from build123d import *

# Parameters (mm, degrees)
F0_W     = 80
F0_H     = 19
F1_DEPTH = 19
F2_R     = 4
F3_DEPTH = 12
F2_R_2   = 5
F4_DEPTH = 2


with BuildPart() as f1:
    # F0 (on Top) → F1 (new body)
    with BuildSketch(Plane.XY):
        Rectangle(F0_W, F0_H)
    extrude(amount=F1_DEPTH)

    # F2 (on face) → F3 (cut)
    with BuildSketch(Plane(origin=(0, 9.5, 0), x_dir=(-1, 0, 0), z_dir=(0, 1, 0))):
        with Locations((20, 9.5)):
            Circle(F2_R)
        with Locations((-20, 9.5)):
            Circle(F2_R)
    extrude(amount=-F3_DEPTH, mode=Mode.SUBTRACT)

    # F2 (on face) → F4 (cut)
    with BuildSketch(Plane(origin=(0, 9.5, 0), x_dir=(-1, 0, 0), z_dir=(0, 1, 0))):
        with Locations((0, 9.5)):
            Circle(F2_R_2)
    extrude(amount=-F4_DEPTH, mode=Mode.SUBTRACT)


solid = f1.part
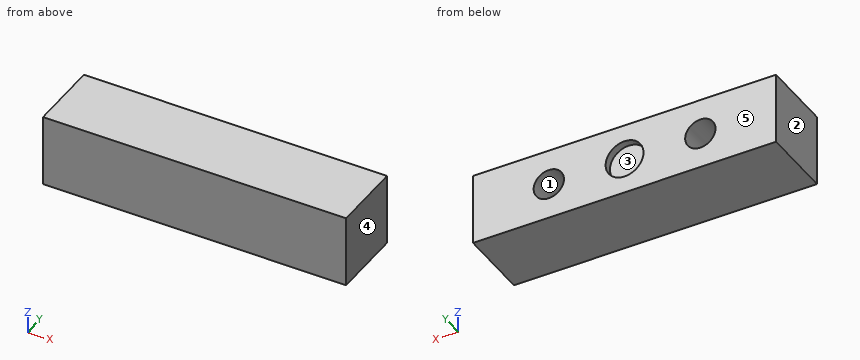
Could you check a few things on this model? Use its own coordinates, in mm. Face numbers are marked on the shaded views. A direction names the side the tool comes from. Give positions to 0.01 mm unless a question says otherwise; leave off trailing zeros. Order: outer loops, then holes, each group sorted by start corner. A loop starts at its lowest first (then second) coordinate and runs counter-clockwise, first axis right, second up.
1. For pin 1 (3 mm diameter, centred on x = -1, z = 10.5, fed in from +Y); pin 2 (10.5 mm diameter, centred on x = 20, z = 9.5, fed in from +Y), each with a flat end and sliding along its axis, tell me the tip position at first contact or that it passes through.
Answers below:
pin 1: stops at y = 7.5
pin 2: stops at y = 9.5
2. Thinking about a two-plate mould opening in X: for the marked faces 3, 4 and 5, which applies, +X half, -X half, draft (parallel to the pull), parting line (faces both ways), or undercut?
Answers below:
face 3: undercut
face 4: +X half
face 5: draft
3. Suppose I cut it at A-A (y = 1.25). Write out the boundary of the cut face in (x, z), plus the area to 3 significant figures.
Answers below:
outline: (-40, 0) - (40, 0) - (40, 19) - (-40, 19) - close; hole circle Ø8 at (-20, 9.5); hole circle Ø8 at (20, 9.5)
area: 1,420 mm2
4. Suppose I cut it at D-D (x = 20). Write out the boundary of the cut face in (y, z).
Answers below:
outline: (-9.5, 0) - (9.5, 0) - (9.5, 5.5) - (-2.5, 5.5) - (-2.5, 13.5) - (9.5, 13.5) - (9.5, 19) - (-9.5, 19) - close
5. Suppose I cut it at C-C (x = 0). Write out the boundary of the cut face in (y, z), plus the area to 3 significant figures.
Answers below:
outline: (-9.5, 0) - (9.5, 0) - (9.5, 4.5) - (7.5, 4.5) - (7.5, 14.5) - (9.5, 14.5) - (9.5, 19) - (-9.5, 19) - close
area: 341 mm2
6. Suppose I cut it at B-B (z = 9.5). Write out the boundary of the cut face in (x, y).
Answers below:
outline: (-40, -9.5) - (40, -9.5) - (40, 9.5) - (24, 9.5) - (24, -2.5) - (16, -2.5) - (16, 9.5) - (5, 9.5) - (5, 7.5) - (-5, 7.5) - (-5, 9.5) - (-16, 9.5) - (-16, -2.5) - (-24, -2.5) - (-24, 9.5) - (-40, 9.5) - close
7. I need wall thicknesses on L1, parallel to X at y = 8, z = 9.75; L2, parallel to Z at x = 20, y = 2.5; L3, parallel to Z at x = 0, y = 8.85. Which ranges of each line are inside material? Lowest first, please.
Answers below:
L1: x = -40 to -23.99, -16.01 to -4.99, 4.99 to 16.01, 23.99 to 40
L2: z = 0 to 5.5, 13.5 to 19
L3: z = 0 to 4.5, 14.5 to 19
8. Which directions (+Z, -Z, +X, -X, +Y, -Y) give clear straight access to the entire face, cutting with the end or side of a thin tool? Please do the marked faces 1 and 2.
Answers below:
face 1: +Y
face 2: +Z, -Z, -X, +Y, -Y
